Autodesk Inventor part; units mm, degrees
ref_plane "YZ Plane" through (0, 0, 0) normal (1, 0, 0) x (0, 1, 0)
ref_plane "XZ Plane" through (0, 0, 0) normal (0, 1, 0) x (-1, 0, 0)
ref_plane "XY Plane" through (0, 0, 0) normal (0, 0, 1) x (1, 0, 0)
sketch "Sketch1" plane through (0, 0, 0) normal (0, 0, 1) x (1, 0, 0)
  line L0 (-117, -19) -> (117, -19)
  line L1 (117, -19) -> (117, 19)
  line L2 (117, 19) -> (-117, 19)
  line L3 (-117, 19) -> (-117, -19)
  line L4 (-117, -19) -> (117, 19) construction
  line L5 (117, -19) -> (-117, 19) construction
  line L6 (-47.035, -11.93) -> (13.035, -11.93)
  line L7 (13.035, -11.93) -> (13.035, -15)
  line L8 (13.035, -15) -> (-47.035, -15)
  line L9 (-47.035, -15) -> (-47.035, -11.93)
  line L10 (-47.035, -11.93) -> (13.035, -15) construction
  line L11 (13.035, -11.93) -> (-47.035, -15) construction
  point P0 (0, 0)
  point P1 (-17, -13.465)
  dimension "d0" = 38
  dimension "d1" = 234
  dimension "d2" = 100
  dimension "d3" = 3.07
  dimension "d4" = 4
  dimension "d5" = 60.07
extrude "Plate1" add sketch "Sketch1" along normal blind 3
sketch "Sketch2" plane through (0, 0, 3) normal (0, 0, 1) x (1, 0, 0)
  line L0 (-84.5251, 6.0599) -> (-93.0599, -2.4749)
  line L1 (-93.0599, -2.4749) -> (-89.4749, -6.0599)
  line L2 (-89.4749, -6.0599) -> (-80.9401, 2.4749)
  line L3 (-80.9401, 2.4749) -> (-84.5251, 6.0599)
  line L4 (-89.4749, 6.0599) -> (-93.0599, 2.4749)
  line L5 (-93.0599, 2.4749) -> (-84.5251, -6.0599)
  line L6 (-84.5251, -6.0599) -> (-80.9401, -2.4749)
  line L7 (-80.9401, -2.4749) -> (-89.4749, 6.0599)
  line L8 (-82.7326, 4.2674) -> (-91.2674, -4.2674)
  line L9 (-91.2674, 4.2674) -> (-82.7326, -4.2674)
  line L10 (-117, 19) -> (-117, -19)
  line L11 (-117, 0) -> (0, 0)
  line L12 (-117, -19) -> (-117, 19)
  point P0 (-87, 0)
  point P1 (-87, -3.585)
  point P2 (-83.415, 0)
  point P3 (-87, 3.585)
  point P4 (-90.585, 0)
  dimension "d7" = 5.07
  dimension "d8" = 30
  dimension "d9" = 12.07
  dimension "d11" = 45
extrude "Cut1" cut sketch "Sketch2" against normal blind 3
pattern_linear "Rectangular Pattern1" count 6 spacing 25 along (1, 0, 0) of "Cut1"
equation "\"d12\" = Thickness"
equation "\"d6\" = Thickness"
equation "\"BendRadius\" = Thickness"
equation "\"BendReliefWidth\" = Thickness"
equation "\"BendReliefDepth\" = 0.5 * Thickness"
equation "\"CornerReliefSize\" = 4 * Thickness"
equation "\"MinimumRemnant\" = 2 * Thickness"
equation "\"TransitionRadius\" = BendRadius"
equation "\"JacobiRadiusSize\" = BendRadius"
equation "\"GapSize\" = Thickness"
properties part number "Extension .1"
Read the model definition and answer for the solid it produces. Units are mm, in the model's axes. Give positions to 0.01 mm unless a question says otherwise; leave off trailing zeros. Answer in a Markdown table with one row per item. Add a question column.
Item 1: Determine the mould class of faces 1 (the face through (-2, 0, 3)), 2 (the face through (-7.708, 4.242, 1.521)) for opening direction Y: pulls with the +Y half, pulls with the -Y half, needs draft (parallel to the pull), parting line crosses it, or undercut.
Item 2: Find the intervals of material crossed by L1, parallel to Y at x = -10.5, z = 2.55 (3 decimals); L2, parallel to Y at x = -38, z = 0.35 (3 decimals); L3, parallel to X at y = -13.5, z = 1.9 (3 decimals), in increasing order.
Item 3: Section A-A, the plane z = 1.2 is taken. Count the separate pieces of the cut face and the enclosed holes in it, and give its area (3 significant figures).
Recorded:
| question | item | result |
|---|---|---|
| 1 | face 1 | needs draft |
| 1 | face 2 | undercut |
| 2 | L1 | y = -19 to -15, -11.93 to -5.085, 5.085 to 19 |
| 2 | L2 | y = -19 to -15, -11.93 to -4.585, 4.585 to 19 |
| 2 | L3 | x = -117 to -47.035, 13.035 to 117 |
| 3 | separate pieces | 1 |
| 3 | enclosed holes | 7 |
| 3 | area | 8,130 mm2 |
